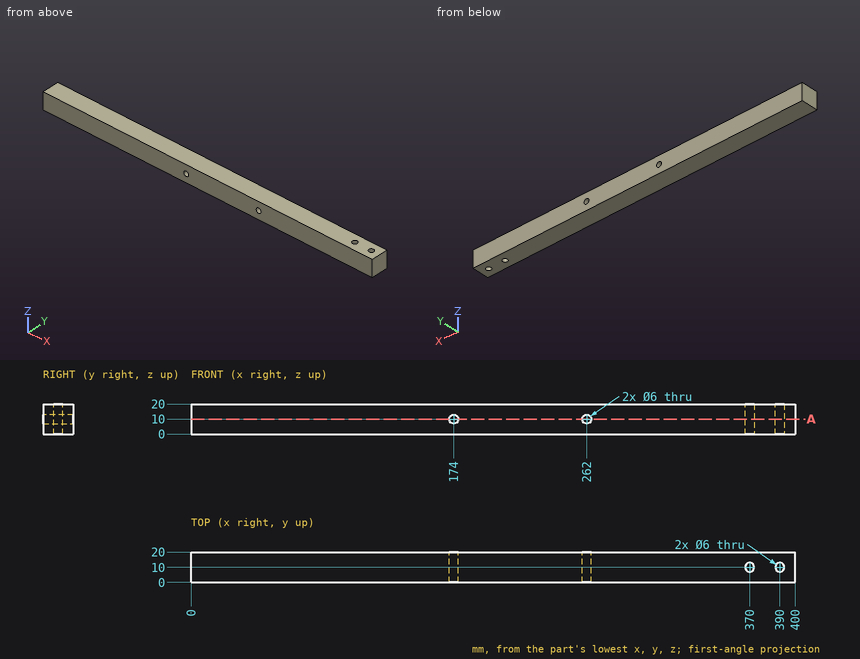
Design review of the part shown in the three views and the two pictorial views. Dimensions are in mm from the part's minimum x, y and z. Give positions to 0.01 mm unless a question says otherwise; leave off trailing zeros. Write each loop counter-clockwise with the first axis right and the second up, starting at its lowest first coordinate (ties: lowest second). Pieces come first, ordered by that corner, then holes. Notation, with made-up numbers: M -13.75,6 L 25.25,6 A19 ccw 25.25,28 Z; hole C 10,-4.75 d11. An arc over 180 degrees is marked long. One line per item, written item: value.
1) For line 1 (Y direction, x = 370, z = 5.75); line 2 (X direction, y = 14.75, z = 7.25); line 3 (X direction, y = 8.5, z = 10), list the stretches that pass through material, from the lowest coordinate up. Write a range as from..to.
Results are:
line 1: y = 0..7, 13..20
line 2: x = 0..172.8, 175.2..260.8, 263.2..400
line 3: x = 0..171, 177..259, 265..367.4, 372.6..387.4, 392.6..400
2) Take a section at A-A, the plane z = 10. Write out the cut boundary in (x, y).
Results are:
outline: M 0,0 L 171,0 L 171,20 L 0,20 Z; M 177,0 L 259,0 L 259,20 L 177,20 Z; M 265,0 L 400,0 L 400,20 L 265,20 Z; hole C 370,10 d6; hole C 390,10 d6
3) For P1, Ø1, axis at x = 47.5, z = 4.5, coming from the -Y side; P2, Ø5.5, axis at x = 390, y = 10, coming from the -Z side, all flat-tipped, find the tip position at first contact; note any pin that passes through.
Results are:
P1: stops at y = 0
P2: passes through
